Source: three-view drawing plus pictorial views. Frame: mm from the lowest corner of the part. A direction names the side the tool comes from. Give positions to 0.01 mm unless a question says otherwise; leave off trailing zeros. Loops run counter-clockwise (first coordinate to the right, second up) from the corner with the lowest first, then second, coordinate; pieces in that order, holes last. Notation, with made-up numbers: M 60,59 L 95,59 A16 ccw 95,66 Z; hole C 20,33 d3. An arc over 180 degrees is marked long. Answer as a JSON object with one key per item and string values. Group by question number.
1) Section query A-A on y = 1.2. Return loops of the section in (x, z).
2) Section query B-B on x = 2.75. Count the separate pieces of the cut face and the enclosed holes in it, plus the area to 3 significant figures.
3) Section query D-D on y = 12.75. Return loops of the section in (x, z).
4) Access query for the marked faces 1 and 2. Directions: +Z, -Z, +X, -X, +Y, -Y. A direction counts if a zero-diameter tool reaches every point of the face in a straight line with its end or side. Return the directions, or none.
5) Draft query along Y for the marked faces 3, 4 and 5. Return one class per face: +Y half, -Y half, draft (parallel to the pull), parting line (faces both ways), or undercut.
6) First-contact query: P1, Ø1, axis at y = 2.5, z = 2, coming from the -X side; P2, Ø1.5, axis at x = 4.5, y = 17.5, coming from the +Z side. Flat tips, straight axial feed; report the tip coordinate or a pass-through.
7) Ray query, L1, parallel to Y at x = 4, z = 1.6 (1 decimal); L2, parallel to Z at x = 0.5, y = 18; L3, parallel to X at y = 1, z = 0.85. Return the intervals inside material, ascending.
8) Section query C-C on x = 6. Return loops of the section in (y, z), plus the area to 3 significant figures.
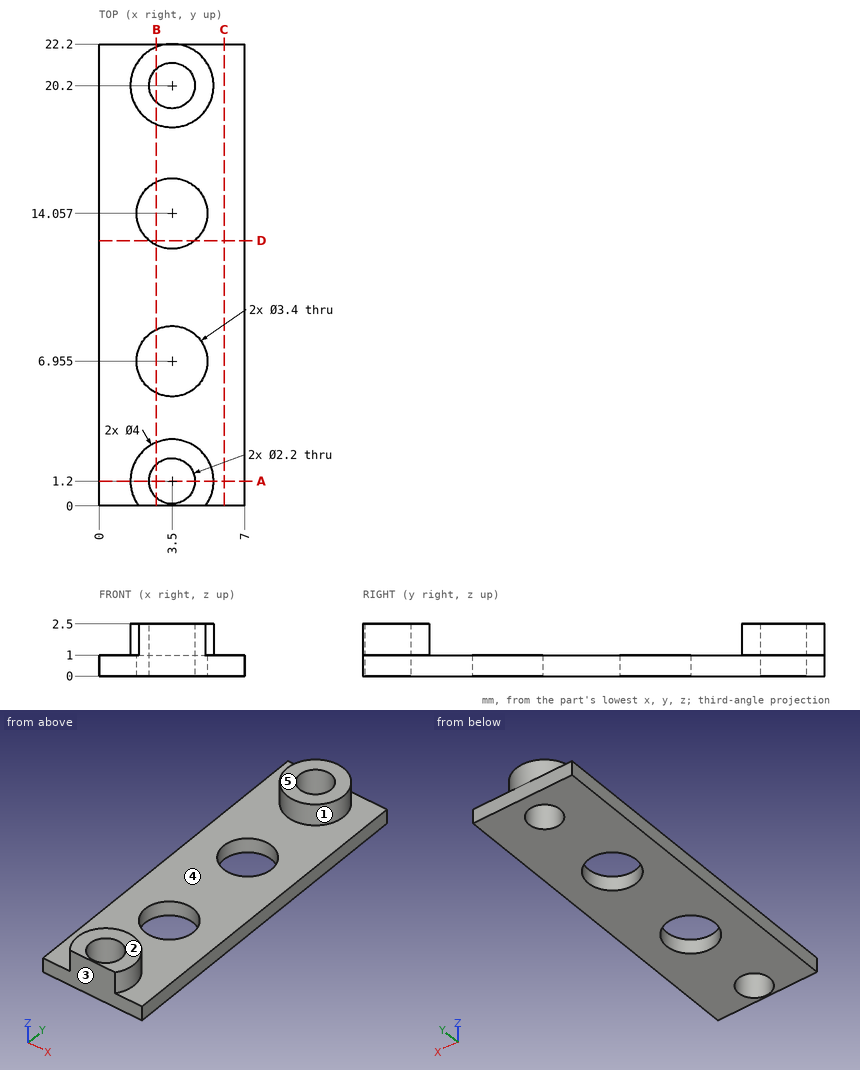
Output:
{
 "1": {"outline": "M 0,0 L 2.4,0 L 2.4,2.5 L 1.5,2.5 L 1.5,1 L 0,1 Z; M 4.6,0 L 7,0 L 7,1 L 5.5,1 L 5.5,2.5 L 4.6,2.5 Z"},
 "2": {"separate pieces": "5", "enclosed holes": "0", "area": "18.2 mm^2"},
 "3": {"outline": "M 0,0 L 2.41,0 L 2.41,1 L 0,1 Z; M 4.59,0 L 7,0 L 7,1 L 4.59,1 Z"},
 "4": {"face 1": "+Z", "face 2": "+Z, +X, -X, +Y, -Y"},
 "5": {"face 3": "-Y half", "face 4": "undercut", "face 5": "draft"},
 "6": {"P1": "stops at x = 1.67", "P2": "stops at z = 1"},
 "7": {"L1": "y = 0 to 0.2, 2.2 to 3.1, 18.3 to 19.2, 21.2 to 22.1", "L2": "z = 0 to 1", "L3": "x = 0 to 2.42, 4.58 to 7"},
 "8": {"outline": "M 0,0 L 22.2,0 L 22.2,1 L 0,1 Z", "area": "22.2 mm^2"}
}
